CAD build for the part. Positions are in the model's coordinates, mm. Face numbers are marked on the shaded views. A direction names the side the tool comes from. Round coordinates to 2 decimals unless told otherwise and drop trailing zeros. Write each loop counter-clockwise with the first axis right and the second up, starting at its lowest first coordinate (ties: lowest second). Pieces come first, ordered by that corner, then holes. Notation, with made-up numbers: (-23.75, 1.25) -> (-2.75, 1.25) arc R30 cw to (-2.75, 26.25) -> close; hole circle Ø10 at (10, 86.5). An arc over 180 degrees is marked (long way). Answer in a Markdown table with one row per item. Add a question column.
```python
from build123d import *

# Parameters (mm, degrees)
BOSS_EXTRUDE1_DEPTH = 30
SKETCH8_W           = 20
SKETCH8_H           = 62.459356161
CUT_EXTRUDE10_DEPTH = 10
SKETCH9_W           = 40
SKETCH9_H           = 57.485293174
CUT_EXTRUDE11_DEPTH = 171.042625644
SKETCH10_W          = 3.787442447
SKETCH10_H          = 24.89779836
CUT_EXTRUDE12_DEPTH = 192.169588314
SKETCH11_R          = 7.5
BOSS_EXTRUDE3_DEPTH = 10
SKETCH13_W          = 7.039311569
SKETCH13_H          = 10
CUT_EXTRUDE13_DEPTH = 14.644416288
CUT_EXTRUDE14_DEPTH = 10
CUT_EXTRUDE15_START = -10
SKETCH15_R          = 7.5
SKETCH15_R_2        = 3.05
CUT_EXTRUDE15_DEPTH = 10
SKETCH16_R          = 2.125
CUT_EXTRUDE16_DEPTH = 192.169588314


with BuildPart() as part:
    # Sketch1 → Boss-Extrude1 (new body)
    with BuildSketch(Plane.XY):
        with BuildLine():
            Line((-13.258302459, -23.24297657), (-8.258302459, -23.24297657))
            Line((-8.258302459, -23.24297657), (-8.258302459, 52.783973791))
            ThreePointArc((-8.258302459, 52.783973791), (-2.701224879, 66.199945851), (10.714747181, 71.75702343))
            Line((10.714747181, 71.75702343), (40.003717522, 71.75702343))
            ThreePointArc((40.003717522, 71.75702343), (48.303722791, 68.31904868), (51.741697541, 60.019043411))
            Line((51.741697541, 60.019043411), (51.741697541, -23.24297657))
            Line((51.741697541, -23.24297657), (54.241697541, -23.24297657))
            Line((54.241697541, -23.24297657), (54.241697541, 0))
            Line((54.241697541, 0), (68.88611383, 0))
            Line((68.88611383, 0), (68.88611383, 10))
            Line((68.88611383, 10), (54.241697541, 10))
            Line((54.241697541, 10), (54.241697541, 71.75702343))
            ThreePointArc((54.241697541, 71.75702343), (50.23063048, 81.422678209), (41.741697541, 87.542446084))
            Line((41.741697541, 87.542446084), (41.741697541, 152.542446084))
            Line((41.741697541, 152.542446084), (-8.258302459, 152.542446084))
            Line((-8.258302459, 152.542446084), (-8.258302459, 83.691556541))
            ThreePointArc((-8.258302459, 83.691556541), (-11.988106196, 74.334235436), (-13.258302459, 64.341363194))
            Line((-13.258302459, 64.341363194), (-13.258302459, -23.24297657))
        make_face()
    extrude(amount=-BOSS_EXTRUDE1_DEPTH)

    # Sketch8 → Cut-Extrude10 (cut)
    with BuildSketch(Plane(origin=(41.741697541, 0, 0), x_dir=(0, 0, -1), z_dir=(1, 0, 0))):
        with Locations((15, 118.812768003)):
            Rectangle(SKETCH8_W, SKETCH8_H)
    extrude(amount=-CUT_EXTRUDE10_DEPTH, mode=Mode.SUBTRACT)

    # Sketch9 → Cut-Extrude11 (cut, through all)
    with BuildSketch(Plane.XY):
        with Locations((16.741697541, 116.299799497)):
            Rectangle(SKETCH9_W, SKETCH9_H)
    extrude(amount=-CUT_EXTRUDE11_DEPTH, mode=Mode.SUBTRACT)

    # Sketch10 → Cut-Extrude12 (cut, through all)
    with BuildSketch(Plane(origin=(0, 152.542446084, 0), x_dir=(1, 0, 0), z_dir=(0, 1, 0))):
        with Locations((12.030722262, 14.765280162)):
            Rectangle(SKETCH10_W, SKETCH10_H)
    extrude(amount=-CUT_EXTRUDE12_DEPTH, mode=Mode.SUBTRACT)

    # Sketch11 → Boss-Extrude3 (add)
    with BuildSketch(Plane.ZY.offset(8.258302459)):
        with Locations(Location((-15.40420704, 109.542446084, 0), (0, 0, 270))):
            Circle(SKETCH11_R)
    extrude(amount=BOSS_EXTRUDE3_DEPTH)

    # Sketch13 → Cut-Extrude13 (cut)
    with BuildSketch(Plane(origin=(68.88611383, 0, 0), x_dir=(0, 0, -1), z_dir=(1, 0, 0))):
        with Locations((14.579402423, 5)):
            Rectangle(SKETCH13_W, SKETCH13_H)
    extrude(amount=-CUT_EXTRUDE13_DEPTH, mode=Mode.SUBTRACT)

    # Sketch14 → Cut-Extrude14 (cut)
    with BuildSketch(Plane(origin=(54.241697541, 0, 0), x_dir=(0, 0, -1), z_dir=(1, 0, 0))):
        with BuildLine():
            ThreePointArc((15, -8.95), (11.95, -12), (15, -15.05))
            Line((15, -15.05), (15, -8.95))
        make_face()
        with BuildLine():
            Line((15, -8.95), (15, -15.05))
            ThreePointArc((15, -15.05), (17.156675683, -14.156675683), (18.05, -12))
            ThreePointArc((18.05, -12), (17.156675683, -9.843324317), (15, -8.95))
        make_face()
    extrude(amount=-CUT_EXTRUDE14_DEPTH, mode=Mode.SUBTRACT)

    # Sketch15 → Cut-Extrude15 (cut)
    # profile 1 of 2: a face of its own
    with BuildSketch(Plane.ZY.offset(13.258302459).offset(CUT_EXTRUDE15_START)):
        with Locations((-15, -12)):
            Circle(SKETCH15_R)
        with Locations(Location((-15, -12, 0), (0, 0, 180))):
            Circle(SKETCH15_R_2, mode=Mode.SUBTRACT)
    # profile 2 of 2: a face of its own
    with BuildSketch(Plane.ZY.offset(13.258302459).offset(CUT_EXTRUDE15_START)):
        with Locations(Location((-15, -12, 0), (0, 0, 180))):
            Circle(SKETCH15_R_2)
    extrude(amount=CUT_EXTRUDE15_DEPTH, mode=Mode.SUBTRACT)

    # Sketch16 → Cut-Extrude16 (cut, through all)
    with BuildSketch(Plane(origin=(0, 152.542446084, 0), x_dir=(1, 0, 0), z_dir=(0, 1, 0))):
        with Locations(Location((1.873560728, 14.765280162, 0), (0, 0, 270))):
            Circle(SKETCH16_R)
    extrude(amount=-CUT_EXTRUDE16_DEPTH, mode=Mode.SUBTRACT)


solid = part.part
```
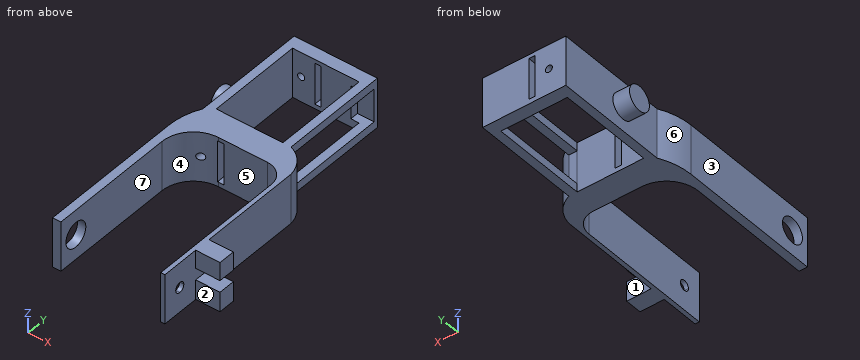
Item 1: Saw through at A-A on x = 57. Give the cut face in (y, z), then the cut area to 3 significant figures.
Item 2: Pin check, flat tips, straight feed: pin 1 (6 mm diameter, centred on y = 150, z = -13.5, fed in from -X); pin 2 (2 mm diameter, centred on y = 148.5, z = -15.5, fed in from +X); pin 3 (1.5 mm diameter, centred on x = 29, z = -25.5, fed in from -Y); pin 4 (2 mm diameter, centred on x = 11.5, z = -24, fed in from -Y). Stop position of each tip, or through.
Item 3: Saw through at C-C on x = 44. Give the cut face in (y, z), then the cut area to 3 significant figures.
Item 4: Saw through at B-B on y = 106. Give the cut face in (x, z).
Item 5: Two-plate mould, pull along Y, no slides. Class the marked faces 5, 6 and 7: +Y half, -Y half, draft (parallel to the pull), parting line (faces both ways), or undercut.
Item 6: Drill centre lines: probe 1 along Y at (x, z) = (20.5, -2); probe 2 along X at (y, z) = (48.5, -6); probe 3 along Y at (x, z) = (-10, -15). Where is each one in solid material? Low to high.
Item 7: Tool access for the marked faces 1, 2, 3 and 4: list every direction of +Z, -Z, +X, -X, +Y, -Y with a clear straight run to the whole face (end or side of a thin tool).
Recorded:
| question | item | result |
|---|---|---|
| 1 | outline | (0, -30) -> (10, -30) -> (10, -18.1) -> (0, -18.1) -> close; (0, -11.06) -> (10, -11.06) -> (10, 0) -> (0, 0) -> close |
| 1 | area | 230 mm2 |
| 2 | pin 1 | x = -8.26 |
| 2 | pin 2 | x = 31.74 |
| 2 | pin 3 | y = 71.76 |
| 2 | pin 4 | through |
| 3 | outline | (71.06, -30) -> (86.55, -30) -> (86.55, 0) -> (71.06, 0) -> close |
| 3 | area | 465 mm2 |
| 4 | outline | (-18.26, -22.01) -> (-8.26, -22.01) -> (-8.26, -30) -> (-3.26, -30) -> (-3.26, 0) -> (-8.26, 0) -> (-8.26, -8.79) -> (-18.26, -8.79) -> close; (36.74, -30) -> (41.74, -30) -> (41.74, -25) -> (36.74, -25) -> close; (36.74, -5) -> (41.74, -5) -> (41.74, 0) -> (36.74, 0) -> close |
| 5 | face 5 | -Y half |
| 5 | face 6 | undercut |
| 5 | face 7 | draft |
| 6 | probe 1 | 71.76 to 87.56, 145.04 to 152.54 |
| 6 | probe 2 | -13.26 to -8.26, 51.74 to 54.24 |
| 6 | probe 3 | -23.24 to -19.5, -4.5 to 80.14, 102.05 to 117.03 |
| 7 | face 1 | +Z, -Z, +X, +Y |
| 7 | face 2 | +Z, -Z, +X, -Y |
| 7 | face 3 | +Z, -Z, -X, -Y |
| 7 | face 4 | +Z, -Z, -Y |
